Work out the finished part from the listing and answer in its coordinate system (mm). A direction names the side the tool comes from. Coordinates: 2 decimals unless noted, no trailing zeros. Order: outer loops, then holes, each group sorted by start corner. A loop starts at its lowest first (then second) coordinate and runs counter-clockwise, first axis right, second up. Notation, with made-up numbers: M -21.75,26 L -4.75,26 A16 ccw -4.75,55 Z; hole C -11.75,40 d10. An arc over 180 degrees is marked long. Answer in a Markdown table with one row per item. Add a question column.
Item 1: Which of the six approach directions +Z, -Z, +X, -X, +Y, -Y give full straight-line access (tool end or side, diameter ignored) to faces 1 (the face through (4.919, 7.715, 7.12)), 2 (the face through (0.801, 25.988, 2.465))?
Item 2: The part is cut by section B-B (x = 0). Write down the section's boundary in (y, z), then the cut area to 3 significant figures.
Item 3: The part is cut by section D-D (z = 6.5). Write down the section's boundary in (x, y), then the cut area to 3 significant figures.
Item 4: Consider line 1 (Z direction, x = 9, y = 9); line 2 (Y direction, x = 4.5, z = 8.75); line 3 (X direction, y = -7, z = 6.25). Determine where each line is inside the solid, lowest interval first. Write a range as from..to.
Item 5: Flat-ended cylindrical pins translate along their axes: pin 1 Ø3 at (y, z) = (21, 3) entering from +X; pin 2 Ø2 at (x, z) = (-17.5, 6.5) entering from -Y; pin 3 Ø5 at (y, z) = (20, 3.5) entering from +X; pin 4 Ø1.5 at (x, y) = (-10.5, 21.5) entering from +Z. Find the tip coordinate at first contact, or state that the pin passes through.
Item 6: The part is cut by section A-A (y = 0). Write down the section's boundary in (x, z).
Item 7: The part is cut by section C-C (z = 3.5). Write down the section's boundary in (x, y), then the cut area to 3 significant figures.
from build123d import *

# Parameters (mm, degrees)
BOSS_EXTRUDE1_DEPTH = 5
SKETCH2_R           = 9.15
BOSS_EXTRUDE2_DEPTH = 4.3


with BuildPart() as part:
    # Sketch1 → Boss-Extrude1 (new body)
    with BuildSketch(Plane.XY):
        with BuildLine():
            Line((-21.021655501, -15.3), (21.021655501, -15.3))
            ThreePointArc((21.021655501, -15.3), (0, 26), (-21.021655501, -15.3))
        make_face()
    extrude(amount=BOSS_EXTRUDE1_DEPTH)

    # Sketch2 → Boss-Extrude2 (add)
    with BuildSketch(Plane.XY.offset(5)):
        Circle(SKETCH2_R)
    extrude(amount=BOSS_EXTRUDE2_DEPTH)

    # Sketch3 → Cut-Revolve1 (revolve, cut)
    with BuildSketch(Plane.XZ):
        with BuildLine():
            Line((0, 9.3), (0, 8.631303449))
            ThreePointArc((0, 8.631303449), (4.088693406, 8.798757997), (8.15, 9.3))
            Line((8.15, 9.3), (0, 9.3))
        make_face()
    revolve(axis=Axis((0, 0, 9.3), (0, 0, -1)), mode=Mode.SUBTRACT)


solid = part.part
Reply:
| question | item | result |
|---|---|---|
| 1 | face 1 | +Z |
| 1 | face 2 | +Z, -Z |
| 2 | outline | M -15.3,0 L 26,0 L 26,5 L 9.15,5 L 9.15,9.3 L 8.15,9.3 A50 cw -8.15,9.3 L -9.15,9.3 L -9.15,5 L -15.3,5 Z |
| 2 | area | 278 mm2 |
| 3 | outline | C 0,0 d18.3 |
| 3 | area | 263 mm2 |
| 4 | line 1 | z = 0..5 |
| 4 | line 2 | y = -7.97..7.97 |
| 4 | line 3 | x = -5.89..5.89 |
| 5 | pin 1 | stops at x = 17.2 |
| 5 | pin 2 | passes through |
| 5 | pin 3 | stops at x = 19.23 |
| 5 | pin 4 | stops at z = 5 |
| 6 | outline | M -26,0 L 26,0 L 26,5 L 9.15,5 L 9.15,9.3 L 8.15,9.3 A50 cw -8.15,9.3 L -9.15,9.3 L -9.15,5 L -26,5 Z |
| 7 | outline | M -21.02,-15.3 L 21.02,-15.3 A26 ccw long Z |
| 7 | area | 1,810 mm2 |
